CAD build for the part. Positions are in the model's coordinates, mm. Round coordinates to 2 decimals unless told otherwise and drop trailing zeros. Loops run counter-clockwise (first coordinate to the right, second up) from the corner with the lowest first, then second, coordinate; pieces in that order, holes last.
```python
from build123d import *

# Parameters (mm, degrees)
ESQUISSE1_R             = 1
BOSS_EXTRU_1_DEPTH      = 5
ESQUISSE2_R             = 3
ENL_V_MAT_EXTRU_1_DEPTH = 2
BOSS_EXTRU_2_START      = 3
ESQUISSE3_R             = 10
ESQUISSE3_R_2           = 3
BOSS_EXTRU_2_DEPTH      = 3
CHANFREIN1_SIZE         = 3


with BuildPart() as part:
    # Esquisse1 → Boss.-Extru.1 (new body)
    with BuildSketch(Plane(origin=(0, 0, 0), x_dir=(0, 0, -1), z_dir=(1, 0, 0))):
        with BuildLine():
            ThreePointArc((20, 0), (0, 20), (-20, 0))
            add(Edge.make_bspline(
                [(-56.568542495, -220), (19.779297851, -184.881212826), (-13.461804543, -52.728965786), (-20, 0)],
                knots=[0, 0, 0, 0, 1, 1, 1, 1], degree=3))
            ThreePointArc((-56.568542495, -220), (0, -260), (56.568542495, -220))
            add(Edge.make_bspline(
                [(56.568542495, -220), (-20.766043456, -183.938290331), (14.228843578, -53.461939266), (20, 0)],
                knots=[0, 0, 0, 0, 1, 1, 1, 1], degree=3))
        make_face()
        Circle(ESQUISSE1_R, mode=Mode.SUBTRACT)
        with BuildLine():
            Line((45, -225), (0, -175))
            Line((0, -175), (-45, -225))
            ThreePointArc((-45, -225), (0, -251.478150705), (45, -225))
        make_face(mode=Mode.SUBTRACT)
        Polygon((-10, -15), (10, -15), (0, -75), align=None, mode=Mode.SUBTRACT)
    extrude(amount=BOSS_EXTRU_1_DEPTH)

    # Esquisse2 → Enlèv. mat.-Extru.1 (cut)
    with BuildSketch(Plane.ZY):
        Circle(ESQUISSE2_R)
    extrude(amount=-ENL_V_MAT_EXTRU_1_DEPTH, mode=Mode.SUBTRACT)

    # Esquisse3 → Boss.-Extru.2 (add)
    with BuildSketch(Plane.ZY.offset(BOSS_EXTRU_2_START)):
        Circle(ESQUISSE3_R)
        Circle(ESQUISSE3_R_2, mode=Mode.SUBTRACT)
    extrude(amount=-BOSS_EXTRU_2_DEPTH)

    # Chanfrein1
    chanfrein1_edges = [part.edges().sort_by_distance(p)[0] for p in [
        (-3, 0, -10),
    ]]
    chamfer(chanfrein1_edges, length=CHANFREIN1_SIZE - 0.0001)  # a hair under: the kernel refuses the full size


solid = part.part
```
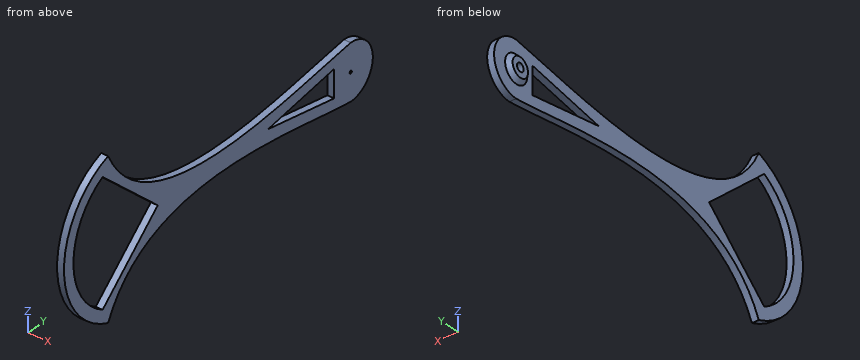
Item 1: Probe line 1 (Y direction, x = -1.3, z = 0); line 2 (Z direction, x = 3.5, y = -208); line 3 (X direction, y = -46, z = 6.5). List the from-to ranges inside material, lowest first.
Answers follow:
line 1: y = -8.7 to -3, 3 to 8.7
line 2: z = -38.21 to -29.7, 29.7 to 38.19
line 3: x = 0 to 5
Item 2: Cut at B-B, the plane x = -1.25. Give the cut face in (y, z).
Answers follow:
outline: circle Ø17.5 at (0, 0); hole circle Ø6 at (0, 0)
Item 3: Cut at A-A, the plane z = 17. State how many separate pieces and enclosed holes the cut face has, plus the area to 3 significant figures.
Answers follow:
separate pieces: 3
enclosed holes: 0
area: 287 mm2
Item 4: Flat gauge pins, fed straight in: P1, Ø4, axis at x = -1, y = -170, coming from the +Z side; P2, Ø2.5, axis at x = 1.5, z = 2.5, coming from the -Y side; P3, Ø1.8, axis at y = 0.5, z = -1.5, coming from the -X side; P4, Ø8, axis at y = -131, z = 14, coming from the +X side. Where does each tip first touch, or does it go through?
Answers follow:
P1: stops at z = 15.28
P2: stops at y = -259.99
P3: stops at x = 2
P4: passes through
